For this review, take the finished solid that the model builds, in its own axes (mm). A direction names the side the tool comes from. Coordinates: 2 decimals unless noted, no trailing zeros. Write each loop counter-clockwise with the first axis right and the second up, starting at its lowest first coordinate (ties: lowest second). Pieces come first, ordered by that corner, then holes.
1) We need section D-D on z = -3. Write out the cut boundary in (x, y).
2) For faces 4 (the face through (16.416, -2.207, -0.054)), 5 (the face through (2, -0.75, 3)), 6 (the face through (12, 2.1, 0)), list the 3-axis set-ups (+Z, -Z, +X, -X, +Y, -Y) from which the entire face can be reached by the end or side of a thin tool; tool diameter is ignored.
3) We need section A-A on x = 12.5. Write out the cut boundary in (y, z), then the cut area to 3 significant figures.
4) Insertion check: P1, Ø2, axis at y = 0, z = -0.5, coming from the +X side; P2, Ø1.3, axis at x = 10.5, z = 3, coming from the +Y side; P3, Ø0.8, axis at x = 3.5, z = 2, coming from the -Y side; P4, Ø2, axis at x = 2, z = 3, coming from the +Y side. Each pin has a flat end and moves straight along its axis. Give the tip position at first contact, or say it passes through.
5) To check wall thickness, follow line 1 along Y through (x, z) = (3, 0); line 2 along Y through (x, z) = (13, 0); line 3 along Z through (x, y) = (8.5, -1.25). State the ranges of each line that lie inside material, in increasing order.
6) Mouldability with a two-part tool opening along Y and no side actions: class faces 1 (the face through (0, 0, -2)), 2 (the face through (19.337, 2.852, -0.048)), 3 (the face through (11, -1.1, 2)) as pulls with the +Y half, pulls with the -Y half, needs draft (parallel to the pull), parting line crosses it, or undercut.
7) We need section C-C on y = -0.25. Write out the cut boundary in (x, z).
8) We need section B-B on z = -0.75. Write out the cut boundary in (x, y), then the cut area to 3 significant figures.
Autodesk Inventor part; units mm, degrees
ref_plane "YZ Plane" through (0, 0, 0) normal (1, 0, 0) x (0, 1, 0)
ref_plane "XZ Plane" through (0, 0, 0) normal (0, 1, 0) x (-1, 0, 0)
ref_plane "XY Plane" through (0, 0, 0) normal (0, 0, 1) x (1, 0, 0)
sketch "Sketch1" plane through (0, 0, 0) normal (1, 0, 0) x (0, 1, 0)
  circle A0 centre (0, 0) radius 4
  dimension "d0" = 8
extrude "Extrusion1" add sketch "Sketch1" along normal blind 20
sketch "Sketch2" plane through (20, 0, 0) normal (1, 0, 0) x (0, 0, -1)
  line L0 (-4, 2.1) -> (4, 2.1)
  line L1 (4, 2.1) -> (4, -1.1)
  line L2 (4, -1.1) -> (-4, -1.1)
  line L3 (-4, -1.1) -> (-4, 2.1)
  point P0 (0, 0)
  dimension "d3" = 8
  dimension "d4" = 3.2
  dimension "d5" = 2.1
  dimension "d6" = 4
extrude "Extrusion2" cut sketch "Sketch2" against normal blind 15
sketch "Sketch3" plane through (0, 0, 0) normal (-1, 0, 0) x (0, 0, 1)
  circle A0 centre (0, 0) radius 1.6
  dimension "d9" = 3.2
extrude "Extrusion3" cut sketch "Sketch3" against normal through all
sketch "Sketch4" plane through (0, 0, 0) normal (0, 0, 1) x (1, 0, 0)
  line L0 (20, 2.1) -> (20, 4)
  line L1 (20, 4) -> (15.3812, -4)
  line L2 (0, -4) -> (20, -4)
  line L3 (20, 4) -> (29.2376, 4) construction
  line L4 (15.3812, -4) -> (20, -4)
  line L5 (20, 4) -> (20, -4)
  point P0 (0, 0)
  dimension "d12" = 120
extrude "Extrusion4" cut sketch "Sketch4" along normal through all both and the other way through all
sketch "Sketch6" plane through (0, 0, 0) normal (-1, 0, 0) x (0, 0, 1)
  line L0 (4, 0.75) -> (1.2, 0.75)
  line L1 (1.2, 0.75) -> (1.2, -0.75)
  line L2 (1.2, -0.75) -> (4, -0.75)
  line L3 (4, -0.75) -> (4, 0.75)
  point P0 (0, 0)
  dimension "d23" = 1.5
  dimension "d24" = 4
  dimension "d25" = 0.75
  dimension "d27" = 1.2
extrude "Extrusion6" cut sketch "Sketch6" against normal blind 10
properties part number "Main_tip_coupler"
Result:
1. outline: (0, -2.65) - (16.16, -2.65) - (17.06, -1.1) - (5, -1.1) - (5, 2.1) - (18.9, 2.1) - (19.22, 2.65) - (0, 2.65) - close
2. face 4: +Z, -Z, +X, -Y
2. face 5: +Z, +X, -X
2. face 6: +Z, -Z, +X
3. outline: (-1.1, -3.85) - (-1.1, -1.16) arc R1.6 cw to (-1.1, 1.16) - (-1.1, 3.85) arc R4 ccw to start; (2.1, -3.4) arc R4 ccw to (2.1, 3.4) - close
3. area: 24.8 mm2
4. P1: passes through
4. P2: stops at y = 3.24
4. P3: stops at y = -3.67
4. P4: stops at y = 3.46
5. line 1: y = -4 to -1.6, 1.6 to 4
5. line 2: y = -4 to -1.6, 2.1 to 4
5. line 3: z = -3.8 to -1, 1 to 3.8
6. face 1: needs draft
6. face 2: pulls with the -Y half
6. face 3: undercut
7. outline: (0, -3.99) - (5, -3.99) - (5, -1.58) - (0, -1.58) - close
8. outline: (0, -3.93) - (15.42, -3.93) - (16.87, -1.41) - (0, -1.41) - close; (0, 1.41) - (5, 1.41) - (5, 2.1) - (18.9, 2.1) - (19.96, 3.93) - (0, 3.93) - close
8. area: 79.6 mm2
